```python
from build123d import *

# Parameters (mm, degrees)
SKETCH1_R           = 1.4224
BOSS_EXTRUDE1_DEPTH = 1.5875


with BuildPart() as part:
    # Sketch1 → Boss-Extrude1 (new body)
    with BuildSketch(Plane.XY):
        with BuildLine():
            Line((-16.984058744, 5.5245), (-20.871224203, 5.5245))
            ThreePointArc((-20.871224203, 5.5245), (21.59, 0), (-20.871224203, -5.5245))
            Line((-20.871224203, -5.5245), (-16.984058744, -5.5245))
            Line((-16.984058744, -5.5245), (-16.984058744, 5.5245))
        make_face()
        with Locations((0, 18.415)):
            Circle(SKETCH1_R, mode=Mode.SUBTRACT)
        with Locations((0, -18.415)):
            Circle(SKETCH1_R, mode=Mode.SUBTRACT)
        Polygon((9.29005, 13.7033), (2.17805, 13.7033), (2.17805, 10.1473), (-3.46075, 10.1473), (-3.46075, 0.4572), (9.29005, 0.4572), align=None, mode=Mode.SUBTRACT)
    extrude(amount=BOSS_EXTRUDE1_DEPTH)


solid = part.part
```
Verification items for the finished model (mm, model axes). A direction names the side the tool comes from. Round coordinates to 2 decimals unless told otherwise and drop trailing zeros. Loops run counter-clockwise (first coordinate to the right, second up) from the corner with the lowest first, then second, coordinate; pieces in that order, holes last. Notation, with made-up numbers: (-3, 15.5) -> (22, 15.5) arc R20 ccw to (22, 40.5) -> close; hole circle Ø8 at (74.5, -16). An arc over 180 degrees is marked (long way). Answer as a JSON object with one key per item and string values.
Q1. Draft check along X on faces 4 (the cylindrical face through (21.572, 0.871, 0.783)), 5 (the flat face through (-19, -5.524, 1)), 6 (the flat face through (3, 0.457, 1)). Enter one of: pulls with the +X half, pulls with the -X half, needs draft (parallel to the pull), parting line crosses it, or undercut.
Data:
{"face 4": "parting line crosses it", "face 5": "needs draft", "face 6": "undercut"}
Q2. Section check C-C (x = 6.5). Record the boundary of the cut face in (y, z).
Data:
{"outline": "(-20.59, 0) -> (0.46, 0) -> (0.46, 1.59) -> (-20.59, 1.59) -> close; (13.7, 0) -> (20.59, 0) -> (20.59, 1.59) -> (13.7, 1.59) -> close"}
Q3. Access from +Z, -Z, +X, -X, +Y, -Y to the whole of each face (thin tool, end or side, straight path). Record for faces 1 (the flat face through (-19, 5.524, 1)), 2 (the flat face through (2.178, 12, 1)), 3 (the flat face through (1, 0, 0)).
Data:
{"face 1": "+Z, -Z, -X", "face 2": "+Z, -Z", "face 3": "-Z, +X, -X, +Y, -Y"}
Q4. Section check B-B (y = 11.5). Record the boundary of the cut face in (x, z), then the cut area to 3 significant figures.
Data:
{"outline": "(-18.27, 0) -> (2.18, 0) -> (2.18, 1.59) -> (-18.27, 1.59) -> close; (9.29, 0) -> (18.27, 0) -> (18.27, 1.59) -> (9.29, 1.59) -> close", "area": "46.7 mm2"}
Q5. Go/stop test with flat-tipped pins: P1, Ø2.5, axis at x = 0, y = 18.415, coming from the -Z side; P2, Ø0.5, axis at x = 6, z = 0.5, coming from the -Y side; P3, Ø0.5, axis at y = 1.5, z = 0.5, coming from the -X side; P4, Ø0.5, axis at x = -1, z = 1, coming from the -Y side. Record where each tip stops, or that it passes through.
Data:
{"P1": "passes through", "P2": "stops at y = -20.81", "P3": "stops at x = -16.98", "P4": "stops at y = -21.58"}
Q6. Section check A-A (x = 0). Record the boundary of the cut face in (y, z).
Data:
{"outline": "(-21.59, 0) -> (-19.84, 0) -> (-19.84, 1.59) -> (-21.59, 1.59) -> close; (-16.99, 0) -> (0.46, 0) -> (0.46, 1.59) -> (-16.99, 1.59) -> close; (10.15, 0) -> (16.99, 0) -> (16.99, 1.59) -> (10.15, 1.59) -> close; (19.84, 0) -> (21.59, 0) -> (21.59, 1.59) -> (19.84, 1.59) -> close"}
Q7. Section check D-D (z = 0.5). Record the boundary of the cut face in (x, y) (1 decimal), then the cut area to 3 significant figures.
Data:
{"outline": "(-20.9, -5.5) arc R21.6 ccw (long way) to (-20.9, 5.5) -> (-17, 5.5) -> (-17, -5.5) -> close; hole (-3.5, 0.5) -> (9.3, 0.5) -> (9.3, 13.7) -> (2.2, 13.7) -> (2.2, 10.1) -> (-3.5, 10.1) -> close; hole circle Ø2.8 at (0, -18.4); hole circle Ø2.8 at (0, 18.4)", "area": "1,250 mm2"}
Q8. Scan lines: line 1 (Y direction, x = 0, z = 0.7); line 2 (X direction, y = 0.5, z = 0.3); line 3 (X direction, y = 18.5, z = 1.2). Record each from-to range of solid material in increasing order. Write a range as from..to.
Data:
{"line 1": "y = -21.59..-19.84, -16.99..0.46, 10.15..16.99, 19.84..21.59", "line 2": "x = -16.98..-3.46, 9.29..21.58", "line 3": "x = -11.13..-1.42, 1.42..11.13"}
